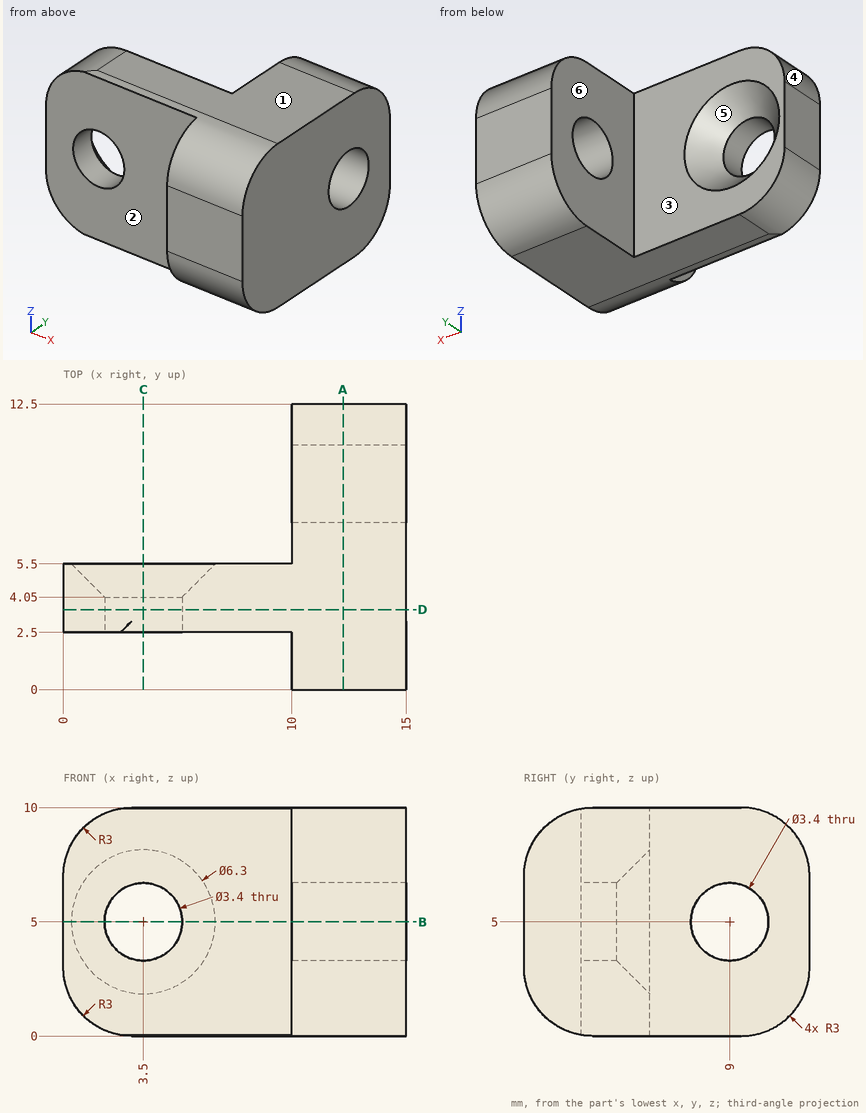
Verification items for this drawing (mm, ordinates from the low corner). A direction names the side the tool comes from. Give positions to 0.01 mm unless a question says otherwise; leave off trailing zeros. Loops run counter-clockwise (first coordinate to the right, second up) from the corner with the lowest first, then second, coordinate; pieces in that order, holes last.
1. Cross-section at C-C on x = 3.5. Record the cut outline in (y, z).
Derived:
outline: (2.5, 0.04) arc R3 ccw to (3, 0) - (5.5, 0) - (5.5, 1.85) - (4.05, 3.3) - (2.5, 3.3) - close; (2.5, 6.7) - (4.05, 6.7) - (5.5, 8.15) - (5.5, 10) - (3, 10) arc R3 ccw to (2.5, 9.96) - close
2. Go/stop test with flat-tipped pins: P1, Ø1.5, axis at y = 10, z = 8, coming from the -X side; P2, Ø5, axis at x = 1.5, z = 4, coming from the -Y side. Record where each tip stops, or that it passes through.
Derived:
P1: stops at x = 10
P2: stops at y = 2.5
3. Tool access check on the marked faces 1, 2 and 3. Record the directions out of +Z, -Z, +X, -X, +Y, -Y that give a thin tool (end or side, any length) a straight path to the whole face; none if there is none.
Derived:
face 1: +Z, +X, -X, +Y, -Y
face 2: +Z, -Z, -X, -Y
face 3: +Z, -Z, -X, +Y
4. Release check for a two-part mould opening along Z. For the marked faces 4, 5 and 6 record: +Z half, -Z half, draft (parallel to the pull), parting line (faces both ways), or undercut.
Derived:
face 4: +Z half
face 5: undercut
face 6: draft
5. Cross-section at A-A on x = 12.25. Record the cut outline in (y, z), and give its area (3 significant figures).
Derived:
outline: (0, 3) arc R3 ccw to (3, 0) - (9.5, 0) arc R3 ccw to (12.5, 3) - (12.5, 7) arc R3 ccw to (9.5, 10) - (3, 10) arc R3 ccw to (0, 7) - close; hole circle Ø3.4 at (9, 5)
area: 108 mm2
6. Cross-section at D-D on y = 3.5. Record the cut outline in (x, z).
Derived:
outline: (0, 3) arc R3 ccw to (3, 0) - (15, 0) - (15, 10) - (3, 10) arc R3 ccw to (0, 7) - close; hole circle Ø3.4 at (3.5, 5)
7. Cross-section at B-B on z = 5. Record the cut outline in (x, y), and give its area (3 significant figures).
Derived:
outline: (0, 2.5) - (1.8, 2.5) - (1.8, 4.05) - (0.35, 5.5) - (0, 5.5) - close; (5.2, 2.5) - (10, 2.5) - (10, 0) - (15, 0) - (15, 7.3) - (10, 7.3) - (10, 5.5) - (6.65, 5.5) - (5.2, 4.05) - close; (10, 10.7) - (15, 10.7) - (15, 12.5) - (10, 12.5) - close
area: 63.2 mm2
8. Material ranges on probe 1 along X at (y, z) = (7.5, 7.5); probe 2 along Y at (x, z) = (7.25, 3.25); probe 3 along Z at (x, y) = (13.7, 9), recorded low to high.
Derived:
probe 1: x = 10 to 15
probe 2: y = 2.5 to 5.5
probe 3: z = 0 to 3.3, 6.7 to 10
